```python
from build123d import *

# Parameters (mm, degrees)
SKETCH_1_W          = 12
SKETCH_1_H          = 10
EXTRUDE_1_DEPTH     = 2
CUT_EXTRUDE_1_DEPTH = 2
FILLET_1_R          = 3


with BuildPart() as part:
    # ｽｹｯﾁ1 → ﾎﾞｽ - 押し出し1 (new body)
    with BuildSketch(Plane.XY):
        Polygon((4, 0), (0, 0), (0, -12), (4, -12), (4, -25), (16, -25), (16, 3), (4, 3), align=None)
        with Locations((10, -30)):
            Rectangle(SKETCH_1_W, SKETCH_1_H)
    extrude(amount=EXTRUDE_1_DEPTH)

    # ｽｹｯﾁ2 → ｶｯﾄ - 押し出し1 (cut)
    with BuildSketch(Plane.XY.offset(2)):
        Polygon((11.632823949, -5.570087609), (8.772941266, -5.570087609), (8.772941266, -10.268637818), (7.260776917, -10.268637818), (10.202882607, -14.99997105), (13.144988298, -10.268637818), (11.632823949, -10.268637818), align=None)
    extrude(amount=-CUT_EXTRUDE_1_DEPTH, mode=Mode.SUBTRACT)

    # ﾌｨﾚｯﾄ1
    fillet_1_edges = [part.edges().sort_by_distance(p)[0] for p in [
        (16, 3, 1),
        (16, -35, 1),
    ]]
    fillet(fillet_1_edges, radius=FILLET_1_R)


solid = part.part
```
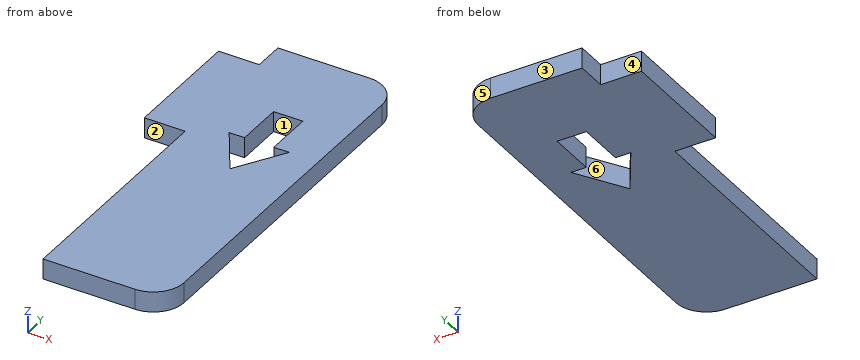
Geometry: final body of the model. Coordinates: model frame, mm. Face numbers are marked on the shaded views. A direction names the side the tool comes from. Coordinates: 2 decimals unless noted, no trailing zeros. Loops run counter-clockwise (first coordinate to the right, second up) from the corner with the lowest first, then second, coordinate; pieces in that order, holes last. Notation, with made-up numbers: (-10, -1.5) -> (24, -1.5) arc R24 cw to (24, 28.5) -> close; hole circle Ø9 at (-21.5, -37.5). An arc over 180 degrees is marked (long way). Use a Markdown table: item, result. Add a question column.
(1) Mould query, pull axis Y, two halves, no side actions, for the marked faces 1, 2 and 3. Classes: pulls with the +Y half, pulls with the -Y half, needs draft (parallel to the pull), parting line crosses it, or undercut.
(2) Section query A-A, the plane y = -7.5. Return loops of the section in (x, z), plus the area to 3 significant figures.
(3) Pin query (flat end, axial travel): pin 1 Ø1 at (y, z) = (-25.5, 0.5) entering from -X. Return the tip coordinate at first contact, or that it passes through.
(4) Section query C-C, the plane x = 12.5. Return loops of the section in (y, z), plus the area to 3 significant figures.
(5) Access query for the marked faces 4, 5 and 6. Directions: +Z, -Z, +X, -X, +Y, -Y. A direction counts if a zero-diameter tool reaches every point of the face in a straight line with its end or side. Return the directions, or none.
(6) Section query B-B, the plane z = 0.5. Return loops of the section in (x, y).
(7) Line query: line 1 along X through (y, z) = (-8.5, 0.8); line 2 along X through (y, z) = (-30, 0.8); line 3 along Y through (x, z) = (2.75, 1). Output: solid intervals per line, ascending.
(8) Section query D-D, the plane x = 3.5. Return loops of the section in (y, z), plus the area to 3 significant figures.
Answer:
| question | item | result |
|---|---|---|
| 1 | face 1 | undercut |
| 1 | face 2 | pulls with the -Y half |
| 1 | face 3 | pulls with the +Y half |
| 2 | outline | (0, 0) -> (8.77, 0) -> (8.77, 2) -> (0, 2) -> close; (11.63, 0) -> (16, 0) -> (16, 2) -> (11.63, 2) -> close |
| 2 | area | 26.3 mm^2 |
| 3 | pin 1 | stops at x = 4 |
| 4 | outline | (-35, 0) -> (-11.31, 0) -> (-11.31, 2) -> (-35, 2) -> close; (-10.27, 0) -> (3, 0) -> (3, 2) -> (-10.27, 2) -> close |
| 4 | area | 73.9 mm^2 |
| 5 | face 4 | +Z, -Z, -X, +Y |
| 5 | face 5 | +Z, -Z, +X, +Y |
| 5 | face 6 | +Z, -Z |
| 6 | outline | (0, -12) -> (4, -12) -> (4, -35) -> (13, -35) arc R3 ccw to (16, -32) -> (16, 0) arc R3 ccw to (13, 3) -> (4, 3) -> (4, 0) -> (0, 0) -> close; hole (7.26, -10.27) -> (10.2, -15) -> (13.14, -10.27) -> (11.63, -10.27) -> (11.63, -5.57) -> (8.77, -5.57) -> (8.77, -10.27) -> close |
| 7 | line 1 | x = 0 to 8.77, 11.63 to 16 |
| 7 | line 2 | x = 4 to 16 |
| 7 | line 3 | y = -12 to 0 |
| 8 | outline | (-12, 0) -> (0, 0) -> (0, 2) -> (-12, 2) -> close |
| 8 | area | 24.0 mm^2 |
